The model under review builds one solid part; all positions refer to its coordinate system, in mm. A direction names the side the tool comes from. Coordinates: 2 decimals unless noted, no trailing zeros. Write each loop counter-clockwise with the first axis right and the second up, starting at its lowest first coordinate (ties: lowest second). Pieces come first, ordered by that corner, then holes.
```python
from build123d import *

# Parameters (mm, degrees)
BOSS_EXTRUDE1_DEPTH = 58
SKETCH5_R           = 3.5
CUT_EXTRUDE3_DEPTH  = 58
SKETCH15_R          = 4
CUT_EXTRUDE4_DEPTH  = 10
SKETCH16_R          = 1.5
CUT_EXTRUDE5_DEPTH  = 10
SKETCH17_R          = 20
SKETCH17_R_2        = 2.5
CUT_EXTRUDE6_DEPTH  = 10


with BuildPart() as part:
    # Sketch2 → Boss-Extrude1 (new body)
    with BuildSketch(Plane.XY):
        Polygon((2, 51.896715462), (36, 51.896715462), (36, -52.603284538), (75.75, -52.603284538), (75.75, -109.603284538), (72.75, -109.603284538), (72.75, -55.603284538), (33, -55.603284538), (33, 48.896715462), (2, 48.896715462), (-29, 48.896715462), (-29, -55.603284538), (-58, -55.603284538), (-58, -109.603284538), (-61, -109.603284538), (-61, -52.603284538), (-32, -52.603284538), (-32, 51.896715462), align=None)
    extrude(amount=BOSS_EXTRUDE1_DEPTH)

    # Sketch5 → Cut-Extrude3 (cut)
    with BuildSketch(Plane.ZY.offset(61)):
        with Locations((29, -96.903284538)):
            Circle(SKETCH5_R)
    extrude(amount=-CUT_EXTRUDE3_DEPTH, mode=Mode.SUBTRACT)

    # Sketch15 → Cut-Extrude4 (cut)
    with BuildSketch(Plane(origin=(75.75, 0, 0), x_dir=(0, 0, -1), z_dir=(1, 0, 0))):
        with Locations((-29, -96.902439923)):
            Circle(SKETCH15_R)
    extrude(amount=-CUT_EXTRUDE4_DEPTH, mode=Mode.SUBTRACT)

    # Sketch16 → Cut-Extrude5 (cut)
    with BuildSketch(Plane(origin=(75.75, 0, 0), x_dir=(0, 0, -1), z_dir=(1, 0, 0))):
        with Locations((-29, -87.402439923)):
            Circle(SKETCH16_R)
        with Locations((-20.772758664, -92.152439923)):
            Circle(SKETCH16_R)
        with Locations((-20.772758664, -101.652439923)):
            Circle(SKETCH16_R)
        with Locations((-29, -106.402439923)):
            Circle(SKETCH16_R)
        with Locations((-37.227241336, -101.652439923)):
            Circle(SKETCH16_R)
        with Locations((-37.227241336, -92.152439923)):
            Circle(SKETCH16_R)
    extrude(amount=-CUT_EXTRUDE5_DEPTH, mode=Mode.SUBTRACT)

    # Sketch17 → Cut-Extrude6 (cut)
    with BuildSketch(Plane(origin=(0, 51.896715462, 0), x_dir=(1, 0, 0), z_dir=(0, 1, 0))):
        with Locations((2, -29)):
            Circle(SKETCH17_R)
        with Locations((-21.5, -5.5)):
            Circle(SKETCH17_R_2)
        with Locations((25.5, -5.5)):
            Circle(SKETCH17_R_2)
        with Locations((25.5, -52.5)):
            Circle(SKETCH17_R_2)
        with Locations((-21.5, -52.5)):
            Circle(SKETCH17_R_2)
    extrude(amount=-CUT_EXTRUDE6_DEPTH, mode=Mode.SUBTRACT)


solid = part.part
```
Item 1: Take a section at D-D, the plane x = 1. Write out the cut boundary in (y, z).
Solved:
outline: (48.9, 0) - (51.9, 0) - (51.9, 9.03) - (48.9, 9.03) - close; (48.9, 48.97) - (51.9, 48.97) - (51.9, 58) - (48.9, 58) - close
Item 2: Take a section at C-C, the plane x = 25.5. Write out the cut boundary in (y, z), plus the area to 3 significant figures.
Solved:
outline: (48.9, 0) - (51.9, 0) - (51.9, 3) - (48.9, 3) - close; (48.9, 8) - (51.9, 8) - (51.9, 50) - (48.9, 50) - close; (48.9, 55) - (51.9, 55) - (51.9, 58) - (48.9, 58) - close
area: 144 mm2
Item 3: Take a section at A-A, the plane z = 5.5. Write out the cut boundary in (x, y), plus the area to 3 significant figures.
Solved:
outline: (-61, -109.6) - (-58, -109.6) - (-58, -55.6) - (-29, -55.6) - (-29, 48.9) - (-24, 48.9) - (-24, 51.9) - (-32, 51.9) - (-32, -52.6) - (-61, -52.6) - close; (-19, 48.9) - (23, 48.9) - (23, 51.9) - (-19, 51.9) - close; (28, 48.9) - (33, 48.9) - (33, -55.6) - (72.75, -55.6) - (72.75, -109.6) - (75.75, -109.6) - (75.75, -52.6) - (36, -52.6) - (36, 51.9) - (28, 51.9) - close
area: 1,330 mm2
Item 4: For pin 1 (5 mm diameter, centred on x = 35.5, y = 22, fed in from -Z); pin 2 (1.8 mm diameter, centred on y = -92.15, z = 37.23, fed in from +X); pin 3 (12 mm diameter, centred on x = 58, z = 36, fed in from -Y); pin 4 (10 mm diameter, centred on y = -13.5, z = 39, fed in from -X), all flat-tipped, find the tip position at first contact; note any pin that passes through.
Solved:
pin 1: stops at z = 0
pin 2: stops at x = -58
pin 3: stops at y = -55.6
pin 4: stops at x = -32
Item 5: Take a section at B-B, the plane y = -76. Write out the cut boundary in (x, z), plus the area to 3 significant figures.
Solved:
outline: (-61, 0) - (-58, 0) - (-58, 58) - (-61, 58) - close; (72.75, 0) - (75.75, 0) - (75.75, 58) - (72.75, 58) - close
area: 348 mm2
Item 6: To check wall thickness, follow line 1 along Z through (x, y) = (25.5, 51.15); line 2 along Y through (x, z) = (73, 29); line 3 along X through (y, z) = (24, 26). State the ranges of each line that lie inside material, in increasing order.
Solved:
line 1: z = 0 to 3, 8 to 50, 55 to 58
line 2: y = -109.6 to -107.9, -104.9 to -100.9, -92.9 to -88.9, -85.9 to -52.6
line 3: x = -32 to -29, 33 to 36
Item 7: Machinability: for faces 4 (the face through (-47, -52.603, 29)), 5 (the face through (53, -55.603, 29)), 6 (the face through (74.271, -92.936, 29.521)), which of the approach directions +Z, -Z, +X, -X, +Y, -Y give a long, thin tool a straight path to every point of the face, cutting with its end or side? Answer none if there is none.
Solved:
face 4: +Z, -Z, -X, +Y
face 5: +Z, -Z, -Y
face 6: +X
Item 8: Mouldability with a two-part tool opening along X and no side actions: class faces 1 (the face through (-61, -82, 29)), 2 (the face through (-59.521, -95.852, 32.338)), 3 (the face through (24.96, 50.42, 54.94)) as pulls with the +X half, pulls with the -X half, needs draft (parallel to the pull), parting line crosses it, or undercut.
Solved:
face 1: pulls with the -X half
face 2: needs draft
face 3: undercut
